Design review of the part built by this model. Coordinates are the model's own, in mm. Face numbers are marked on the shaded views. A direction names the side the tool comes from. Give positions to 0.01 mm unless a question says otherwise; leave off trailing zeros. Order: outer loops, then holes, each group sorted by start corner. A loop starts at its lowest first (then second) coordinate and runs counter-clockwise, first axis right, second up. Notation, with made-up numbers: M -19.75,38 L -3.75,38 A25 ccw -3.75,57 Z; hole C -2.75,1.5 d3. An arc over 180 degrees is marked long. Answer as a JSON object with one key per item and string values.
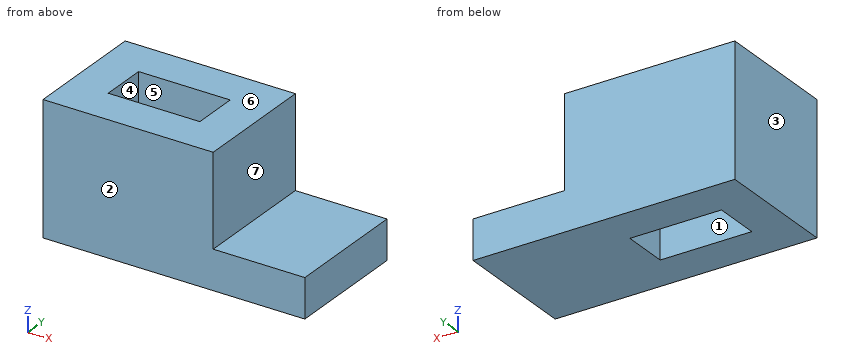
from build123d import *

# Parameters (mm, degrees)
F0_W     = 127
F0_H     = 60.452662
F1_DEPTH = 63.5
F2_W     = 44.45
F2_H     = 22.352662
F3_DEPTH = 63.501
F4_W     = 44.45
F4_H     = 44.45
F5_DEPTH = 63.5


with BuildPart() as f1:
    # F0 (on Top) → F1 (new body)
    with BuildSketch(Plane.XY):
        with Locations((63.5, 30.226331)):
            Rectangle(F0_W, F0_H)
    extrude(amount=F1_DEPTH)

    # F2 (on face) → F3 (cut, through all)
    with BuildSketch(Plane.XY.offset(63.5)):
        with Locations((41.275, 30.226331)):
            Rectangle(F2_W, F2_H)
    extrude(amount=-F3_DEPTH, mode=Mode.SUBTRACT)

    # F4 (on face) → F5 (cut)
    with BuildSketch(Plane.XZ):
        with Locations((104.775, 41.275)):
            Rectangle(F4_W, F4_H)
    extrude(amount=-F5_DEPTH, mode=Mode.SUBTRACT)


solid = f1.part
(1) To check wall thickness, follow L1, parallel to Y at x = 26, z = 8; L2, parallel to X at y = 29.5, z = 42; L3, parallel to X at y = 40.5, z = 16.5. State the ranges of each line that lie inside material, in increasing order. Write a range as from..to.
Checked values:
{"L1": "y = 0..19.05, 41.4..60.45", "L2": "x = 0..19.05, 63.5..82.55", "L3": "x = 0..19.05, 63.5..127"}
(2) We need section A-A (z = 16). Write out the cut boundary in (x, y).
Checked values:
{"outline": "M 0,0 L 127,0 L 127,60.45 L 0,60.45 Z; hole M 19.05,19.05 L 63.5,19.05 L 63.5,41.4 L 19.05,41.4 Z"}
(3) Insertion check: pin 1 (4 mm diameter, centred on y = 51.5, z = 24.5, fed in from +X). The pin has a flat end and moves straight along its axis. Give the tip position at first contact, or say it passes through.
Checked values:
{"pin 1": "stops at x = 82.55"}
(4) Draft analysis for pull direction Y (two halves, no side actions). For the marked faces 1, 2, 3 and 4, state which applies: +Y half, -Y half, draft (parallel to the pull), parting line (faces both ways), or undercut.
Checked values:
{"face 1": "undercut", "face 2": "-Y half", "face 3": "draft", "face 4": "undercut"}
(5) We need section D-D (z = 33). Write out the cut boundary in (x, y).
Checked values:
{"outline": "M 0,0 L 82.55,0 L 82.55,60.45 L 0,60.45 Z; hole M 19.05,19.05 L 63.5,19.05 L 63.5,41.4 L 19.05,41.4 Z"}
(6) We need section C-C (y = 30). Write out the cut boundary in (x, z), plus the area to 3 significant figures.
Checked values:
{"outline": "M 0,0 L 19.05,0 L 19.05,63.5 L 0,63.5 Z; M 63.5,0 L 127,0 L 127,19.05 L 82.55,19.05 L 82.55,63.5 L 63.5,63.5 Z", "area": "3,270 mm^2"}
(7) Tool access review of the marked faces 5, 6 and 7: name each direction out of +Z, -Z, +X, -X, +Y, -Y from which nothing blocks a thin tool from reaching the whole face with its end or side.
Checked values:
{"face 5": "+Z, -Z", "face 6": "+Z, +X, -X, +Y, -Y", "face 7": "+Z, +X, +Y, -Y"}
(8) We need section B-B (x = 47). Write out the cut boundary in (y, z), plus the area to 3 significant figures.
Checked values:
{"outline": "M 0,0 L 19.05,0 L 19.05,63.5 L 0,63.5 Z; M 41.4,0 L 60.45,0 L 60.45,63.5 L 41.4,63.5 Z", "area": "2,420 mm^2"}
